Could you check a few things on this model? Use its own coordinates, in mm. A direction names the side the tool comes from. Give positions to 0.01 mm unless a question says otherwise; leave off trailing zeros. Loops run counter-clockwise (first coordinate to the right, second up) from the corner with the lowest first, then second, coordinate; pieces in that order, holes last.
1. For faces 1 (the flat face through (-0.5, -12.6, 0)), 2 (the flat face through (-24.4, -13, 184)), which set-ups out of +Z, -Z, +X, -X, +Y, -Y let a thin tool reach every point of the face, with its end or its side?
2. Thinking about a two-plate mould opening in X: for faces 3 (the flat face through (-13, -25.4, 178)), 4 (the flat face through (-25.4, -13, 218)), 5 (the flat face through (-1, -13, 178)), which applies, +X half, -X half, draft (parallel to the pull), parting line (faces both ways), or undercut?
3. I need wall thicknesses on line 1 along Y through (x, z) = (-8, 234); line 2 along X through (y, z) = (-20, 329.5). Which ranges of each line are inside material? Lowest first, please.
4. Imagine slicing it at C-C (x = -4.5). List the corners of the cut face in (y, z) for me.
5. For P1, Ø0.8, axis at x = -25, y = -8.5, coming from the -Z side; P2, Ø1.1, axis at x = -25, y = -8.5, coming from the +Z side; P3, Ø12, axis at x = -11, y = -17, coming from the +Z side, each with a flat end and sliding along its axis, tell me the tip position at first contact or that it passes through.
6. Imagine slicing it at A-A (y = -7). List the corners of the cut face in (x, z) for me.
7. Imagine slicing it at D-D (z = 46). List the corners of the cut face in (x, y) for me.
8. Imagine slicing it at B-B (z = 182). List the corners of the cut face in (x, y) for me.
```python
from build123d import *

# Parameters (mm, degrees)
CROQUIS1_W              = 25.4
CROQUIS1_H              = 25.4
CROQUIS1_W_2            = 23.4
CROQUIS1_H_2            = 23.4
SALIENTE_EXTRUIR1_DEPTH = 361
CROQUIS2_W              = 50
CROQUIS2_H              = 23.4
CORTAR_EXTRUIR1_DEPTH   = 1
CORTAR_EXTRUIR2_REACH   = 364.783
CROQUIS3_W              = 11
CROQUIS3_H              = 23.4


with BuildPart() as part:
    # Croquis1 → Saliente-Extruir1 (new body)
    with BuildSketch(Plane.XY):
        with Locations((-12.7, -12.7)):
            Rectangle(CROQUIS1_W, CROQUIS1_H)
        with Locations((-12.7, -12.7)):
            Rectangle(CROQUIS1_W_2, CROQUIS1_H_2, mode=Mode.SUBTRACT)
    extrude(amount=SALIENTE_EXTRUIR1_DEPTH)

    # Croquis2 → Cortar-Extruir1 (cut)
    with BuildSketch(Plane.ZY.offset(25.4)):
        with Locations((336, -12.7)):
            Rectangle(CROQUIS2_W, CROQUIS2_H)
        with Locations((25, -12.7)):
            Rectangle(CROQUIS2_W, CROQUIS2_H)
    extrude(amount=-CORTAR_EXTRUIR1_DEPTH, mode=Mode.SUBTRACT)

    # Croquis3 → Cortar-Extruir2 (cut, up to next)
    with BuildSketch(Plane.ZY.offset(25.4), mode=Mode.PRIVATE) as cortar_extruir2_sk1:
        with Locations((55.5, -12.7)):
            Rectangle(CROQUIS3_W, CROQUIS3_H)
    cortar_extruir2_tool1 = extrude(cortar_extruir2_sk1.sketch, amount=-CORTAR_EXTRUIR2_REACH, mode=Mode.PRIVATE) & part.part
    add(cortar_extruir2_tool1.solids().sort_by_distance((-25.4, -12.7, 55.5))[0], mode=Mode.SUBTRACT)


solid = part.part
```
Derived:
1. face 1: -Z, +X, -X, +Y, -Y
1. face 2: +Z, -Z
2. face 3: draft
2. face 4: -X half
2. face 5: undercut
3. line 1: y = -25.4 to -24.4, -1 to 0
3. line 2: x = -1 to 0
4. outline: (-25.4, 0) - (-24.4, 0) - (-24.4, 361) - (-25.4, 361) - close; (-1, 0) - (0, 0) - (0, 361) - (-1, 361) - close
5. P1: stops at z = 61
5. P2: stops at z = 311
5. P3: passes through
6. outline: (-25.4, 61) - (-24.4, 61) - (-24.4, 311) - (-25.4, 311) - close; (-1, 0) - (0, 0) - (0, 361) - (-1, 361) - close
7. outline: (-25.4, -25.4) - (0, -25.4) - (0, 0) - (-25.4, 0) - (-25.4, -1) - (-1, -1) - (-1, -24.4) - (-25.4, -24.4) - close
8. outline: (-25.4, -25.4) - (0, -25.4) - (0, 0) - (-25.4, 0) - close; hole (-24.4, -24.4) - (-1, -24.4) - (-1, -1) - (-24.4, -1) - close
